Autodesk Fusion 360 part; units mm, degrees
sketch "草图1" plane through (0, 0, 0) normal (0, 0, 1) x (1, 0, 0)
  line L0 (22.5, -15) -> (-22.5, -15)
  line L1 (-22.5, -15) -> (-22.5, 15)
  line L2 (-22.5, 15) -> (22.5, 15)
  line L3 (22.5, 15) -> (22.5, -15)
  line L4 (22.5, -15) -> (-22.5, 15) construction
  line L5 (-22.5, -15) -> (22.5, 15) construction
  dimension "d27" = 45
  dimension "d28" = 30
extrude "拉伸1" add sketch "草图1" along normal blind 8
sketch "草图2" plane through (0, 0, 0) normal (1, 0, 0) x (0, 1, 0)
  circle A0 centre (5, 8) radius 1.8
  dimension "d31" = 3.6
extrude "拉伸2" cut sketch "草图2" along normal blind 12.5 and the other way blind 12.5
mirror "镜像1" about plane through (0, 0, 0) normal (0, 1, 0) of "拉伸2"
sketch "草图3" plane through (0, 0, 8) normal (0, 0, 1) x (-1, 0, 0)
  line L0 (12.5, 6.8) -> (12.5, 3.2)
  line L1 (12.5, 3.2) -> (-12.5, 3.2)
  line L2 (-12.5, 3.2) -> (-12.5, 6.8)
  line L3 (-12.5, 6.8) -> (12.5, 6.8)
  line L4 (12.5, -3.2) -> (12.5, -6.8)
  line L5 (12.5, -6.8) -> (-12.5, -6.8)
  line L6 (-12.5, -6.8) -> (-12.5, -3.2)
  line L7 (-12.5, -3.2) -> (12.5, -3.2)
  line L8 (-22.5, -15) -> (22.5, -15)
  line L9 (22.5, -15) -> (22.5, 15)
  line L10 (22.5, 15) -> (-22.5, 15)
  line L11 (-22.5, 15) -> (-22.5, -15)
  circle A0 centre (17, 10) radius 2
  circle A1 centre (-17, -10) radius 2
  dimension "d38" = 4
  dimension "d39" = 4
extrude "拉伸3" add sketch "草图3" along normal blind 3 contours A0 | A1
fillet "圆角1" radius 2 4 edges at (-22.5, -15, 4) (-22.5, 15, 4) (22.5, 15, 4) (22.5, -15, 4)
equation "Catheter_Diameter = Flexible spring catheter outer diameter"
equation "Catheter_Assembly_Clearance = Initial diametral assembly clearance between catheter and Ecoflex liner"
equation "Clamp_Groove_Diameter = Hard clamp circular groove diameter"
equation "Pad_Outer_Diameter = Ecoflex liner outer diameter driven by clamp groove"
equation "Pad_Outer_Radius = Ecoflex liner outer radius"
equation "Pad_Inner_Diameter = Ecoflex liner inner diameter"
equation "Pad_Inner_Radius = Ecoflex liner inner radius"
equation "Pad_Radial_Thickness = Nominal radial thickness of Ecoflex liner"
equation "Pad_Length = Effective Ecoflex liner length"
equation "Mold_Length = Overall mold length along X"
equation "Mold_Width = Overall mold width along Y"
equation "Bottom_Mold_Thickness = Bottom mold plate thickness"
equation "Top_Mold_Thickness = Top mold plate thickness"
equation "Top_Mold_Base_Z = Assembly Z height of top mold bottom parting face"
equation "Pad_Cavity_Offset_Y = Centerline offset of the two cavities from mold center"
equation "Alignment_Pin_Diameter = Printed alignment pin diameter on bottom mold"
equation "Alignment_Pin_Height = Alignment pin height"
equation "Alignment_Hole_Diameter = Alignment blind-hole diameter on top mold"
equation "Alignment_Hole_Depth = Alignment blind-hole depth"
equation "Alignment_Pin_Offset_X = Absolute X coordinate magnitude of alignment pins"
equation "Alignment_Pin_Offset_Y = Absolute Y coordinate magnitude of alignment pins"
equation "Overflow_Channel_Width = Optional V1 overflow-channel width; retained but not used in recommended V1"
equation "Overflow_Channel_Depth = Optional V1 overflow-channel depth; retained but not used in recommended V1"
equation "Overflow_Well_Diameter = Optional overflow-well diameter; retained but not used in recommended V1"
equation "Overflow_Well_Depth = Optional overflow-well depth; retained but not used in recommended V1"
equation "Mold_Outer_Fillet = External handling-edge fillet radius"
equation "d27 = Mold_Length"
equation "d28 = Mold_Width"
equation "d29 = Bottom_Mold_Thickness"
equation "d31 = Pad_Outer_Diameter"
equation "d32 = Pad_Length / 2"
equation "d34 = Pad_Length / 2"
equation "d38 = Alignment_Pin_Diameter"
equation "d43 = Mold_Outer_Fillet"
Could you check a few things on this model? Use its own coordinates, in mm. A direction names the side the tool comes from. Give positions to 0.01 mm unless a question says otherwise; leave off trailing zeros. Write each loop counter-clockwise with the first axis right and the second up, starting at its lowest first coordinate (ties: lowest second). Pieces come first, ordered by that corner, then holes. Notation, with made-up numbers: (47.5, 25.5) -> (55.5, 25.5) arc R31 cw to (55.5, 50.5) -> close; hole circle Ø2 at (64.25, 78.5). An arc over 180 degrees is marked (long way). Write each question's results on one line, items separated by ' | '. Start each with the question number.
Q1. Suppose I cut it at D-D, the plane z = 6.75. List the corners of the cut face in (x, y) for me, and give its area (3 significant figures).
Q2. Suppose I cut it at B-B, the plane x = -17. List the corners of the cut face in (y, z) for me.
Q3. I'm going to push a flat-ended pin straight in: pin 1 Ø12 at (x, y) = (-6, -4) entering from +Z. Where does the tip first touch, or does it pass through?
Q4. I need wall thicknesses on probe 1 along Z at (x, y) = (-15.5, -13); probe 2 along Z at (x, y) = (-12, -4.5); probe 3 along X at (y, z) = (8.25, 10). Which ranges of each line are inside material? Lowest first, please.
Q5. We'd pull the mould along X, two halves only. Please class faces 1 (the face through (-22.5, 0, 4)), 2 (the face through (21.9, -14.43, 4.06)), 3 (the face through (18.474, 11.352, 9.479)), 4 (the face through (-12.5, -5, 7)): +X half, -X half, draft (parallel to the pull), parting line (faces both ways), or undercut.
Q6. Which directions (+Z, -Z, +X, -X, +Y, -Y) give clear straight access to the entire face, cutting with the end or side of a thin tool? Please do faces 5 (the face through (0.2, 5, 6.2)), 6 (the face through (-17, -10, 11)).
Q7. Suppose I cut it at A-A, the plane z = 10.25. List the corners of the cut face in (x, y) for me.
Q8. Suppose I cut it at C-C, the plane y = 10. List the corners of the cut face in (x, z) for me.
Outcome:
1) outline: (-22.5, -13) arc R2 ccw to (-20.5, -15) -> (20.5, -15) arc R2 ccw to (22.5, -13) -> (22.5, 13) arc R2 ccw to (20.5, 15) -> (-20.5, 15) arc R2 ccw to (-22.5, 13) -> close; hole (-12.5, -6.3) -> (12.5, -6.3) -> (12.5, -3.7) -> (-12.5, -3.7) -> close; hole (-12.5, 3.7) -> (12.5, 3.7) -> (12.5, 6.3) -> (-12.5, 6.3) -> close | area: 1,220 mm2
2) outline: (-15, 0) -> (15, 0) -> (15, 8) -> (-8, 8) -> (-8, 11) -> (-12, 11) -> (-12, 8) -> (-15, 8) -> close
3) pin 1: z = 8
4) probe 1: 0 to 8 | probe 2: 0 to 6.27 | probe 3: 16.03 to 17.97
5) face 1: -X half | face 2: +X half | face 3: parting line | face 4: undercut
6) face 5: +Z | face 6: +Z, +X, -X, +Y, -Y
7) outline: circle Ø4 at (-17, -10); circle Ø4 at (17, 10)
8) outline: (-22.5, 0) -> (22.5, 0) -> (22.5, 8) -> (19, 8) -> (19, 11) -> (15, 11) -> (15, 8) -> (-22.5, 8) -> close
